Geometry check sheet. Reference: drawing and pictorial views, mm from the part's lowest x, y, z. A direction names the side the tool comes from. Coordinates: 2 decimals unless noted, no trailing zeros. Write each loop counter-clockwise with the first axis right and the second up, starting at its lowest first coordinate (ties: lowest second). Pieces come first, ordered by that corner, then holes. Notation, with made-up numbers: (-11.75, -37) -> (33.25, -37) arc R18 ccw to (33.25, -31) -> close; hole circle Ø8 at (-2, 74.5). An arc over 180 degrees is marked (long way). Use a Markdown table: item, result.
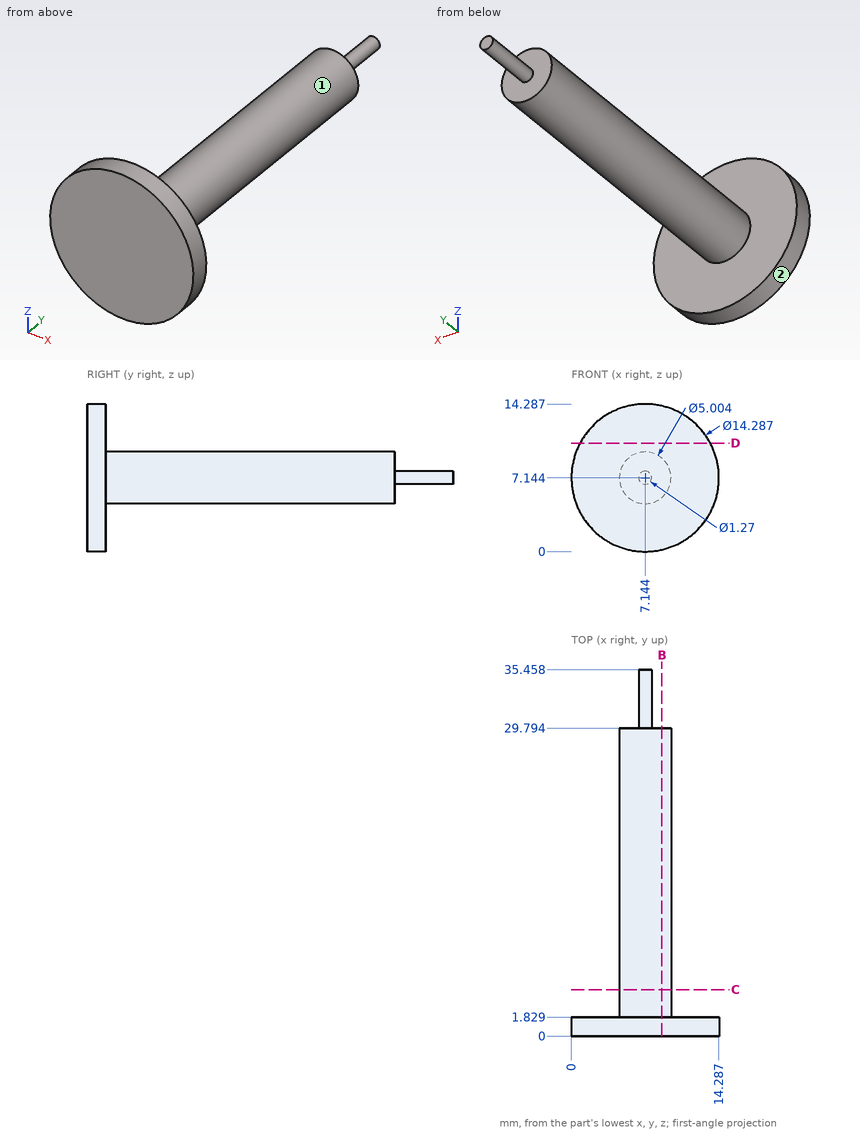
Item 1: Section check D-D on z = 10.5. Record the boundary of the cut face in (x, y).
Answer block:
| item | result |
|---|---|
| outline | (0.84, 0) -> (13.45, 0) -> (13.45, 1.83) -> (0.84, 1.83) -> close |
Item 2: Section check C-C on y = 4.5. Record the boundary of the cut face in (x, z) (1 decimal).
Answer block:
| item | result |
|---|---|
| outline | circle Ø5 at (7.1, 7.1) |
Item 3: Tool access check on the marked faces 1 and 2. Record the directions out of +Z, -Z, +X, -X, +Y, -Y that give a thin tool (end or side, any length) a straight path to the whole face; none if there is none.
Answer block:
| item | result |
|---|---|
| face 1 | +Y |
| face 2 | +Y, -Y |
Item 4: Section check B-B on x = 8.75. Record the boundary of the cut face in (y, z) (1 decimal), then the cut area to 3 significant figures.
Answer block:
| item | result |
|---|---|
| outline | (0, 0.2) -> (1.8, 0.2) -> (1.8, 5.2) -> (29.8, 5.2) -> (29.8, 9.1) -> (1.8, 9.1) -> (1.8, 14.1) -> (0, 14.1) -> close |
| area | 133 mm^2 |
Item 5: Thickness scan on L1, parallel to Y at x = 4, z = 9.25; L2, parallel to Z at x = 7.75, y = 12.5 (1 decimal); L3, parallel to X at y = 15, z = 6. Record the ranges inside material, lowest first. Write a range as [from, to].
Answer block:
| item | result |
|---|---|
| L1 | y = [0, 1.83] |
| L2 | z = [4.7, 9.6] |
| L3 | x = [4.92, 9.37] |
Item 6: Depth check by flat-ended pin: P1, Ø4, axis at y = 21, z = 4, coming from the +X side; P2, Ø4, axis at x = 9, y = 13, coming from the -Z side; P3, Ø4, axis at x = 7, y = 9.5, coming from the +Z side; P4, Ø1.5, axis at y = 7.5, z = 12, coming from the +X side. Enter the tip coordinate at first touch or a pass-through.
Answer block:
| item | result |
|---|---|
| P1 | stops at x = 9.37 |
| P2 | stops at z = 4.64 |
| P3 | stops at z = 9.65 |
| P4 | passes through |
